```python
from build123d import *

# Parameters (mm, degrees)
SKETCH1_W           = 4
SKETCH1_H           = 15
BOSS_EXTRUDE1_DEPTH = 1
SKETCH2_R           = 1.5
CUT_EXTRUDE1_DEPTH  = 0.1
CUT_EXTRUDE2_DEPTH  = 0.2
SKETCH4_R           = 2.849028986
BOSS_EXTRUDE2_DEPTH = 4
CUT_EXTRUDE3_START  = -0.5
CUT_EXTRUDE3_DEPTH  = 3
SKETCH6_R           = 1
CUT_EXTRUDE4_DEPTH  = 50.5
BOSS_EXTRUDE3_REACH = 11.393
SKETCH7_W           = 4
SKETCH7_H           = 0.331547144
SKETCH8_R           = 1.5
BOSS_EXTRUDE4_DEPTH = 1.5
SKETCH13_R          = 2.5
CUT_EXTRUDE6_DEPTH  = 3
SKETCH14_R          = 1.5
BOSS_EXTRUDE5_DEPTH = 1
SKETCH15_R          = 1.65511662
CUT_EXTRUDE7_DEPTH  = 1.5
SKETCH16_W          = 5.099694499
SKETCH16_H          = 2.218752709
CUT_EXTRUDE8_DEPTH  = 3
FILLET1_R           = 0.2
SKETCH17_R          = 1.288740584
BOSS_EXTRUDE6_DEPTH = 1
FILLET2_R           = 1
SKETCH18_R          = 1.986595171
BOSS_EXTRUDE7_DEPTH = 0.5


with BuildPart() as part:
    # Sketch1 → Boss-Extrude1 (new body)
    with BuildSketch(Plane.XY):
        Rectangle(SKETCH1_W, SKETCH1_H)
    extrude(amount=BOSS_EXTRUDE1_DEPTH)

    # Sketch2 → Cut-Extrude1 (cut)
    with BuildSketch(Plane.XY.offset(1)):
        with Locations((0, -5.001272615)):
            Circle(SKETCH2_R)
        with Locations((0, -1.683913286)):
            Circle(SKETCH2_R)
    extrude(amount=-CUT_EXTRUDE1_DEPTH, mode=Mode.SUBTRACT)

    # Sketch3 → Cut-Extrude2 (cut)
    with BuildSketch(Plane.XY.offset(0.9)):
        Polygon((-0.108557852, -6.107102786), (0.108557852, -6.107102786), (0.108557852, -5.098298557), (0.933492592, -5.098298557), (0.933492592, -4.904246673), (0.108557852, -4.904246673), (0.108557852, -3.948637219), (-0.108557852, -3.948637219), (-0.108557852, -4.904246673), (-0.962043741, -4.904246673), (-0.962043741, -5.098298557), (-0.108557852, -5.098298557), align=None)
        Polygon((-0.962043741, -1.780939228), (-0.962043741, -1.586887344), (-0.108557852, -1.586887344), (-0.108557852, -0.578083116), (0.108557852, -0.578083116), (0.108557852, -1.586887344), (0.933492592, -1.586887344), (0.933492592, -1.780939228), (0.108557852, -1.780939228), (0.108557852, -2.736548682), (-0.108557852, -2.736548682), (-0.108557852, -1.780939228), align=None)
    extrude(amount=-CUT_EXTRUDE2_DEPTH, mode=Mode.SUBTRACT)

    # Sketch4 → Boss-Extrude2 (add)
    with BuildSketch(Plane(origin=(2, 0, 0), x_dir=(0, 0, -1), z_dir=(1, 0, 0))):
        with Locations((-2.871998104, 5.020758916)):
            Circle(SKETCH4_R)
    extrude(amount=-BOSS_EXTRUDE2_DEPTH)

    # Sketch5 → Cut-Extrude3 (cut)
    with BuildSketch(Plane(origin=(2, 0, 0), x_dir=(0, 0, -1), z_dir=(1, 0, 0)).offset(CUT_EXTRUDE3_START)):
        with BuildLine():
            Line((-2.871998104, 7.200015745), (-2.871998104, 9.297132531))
            Line((-2.871998104, 9.297132531), (-14.767112772, 7.450442617))
            Line((-14.767112772, 7.450442617), (-10.359701014, 0.939041163))
            Line((-10.359701014, 0.939041163), (-1.261981382, 2.30327176))
            Line((-1.261981382, 2.30327176), (-1.761184463, 3.145858016))
            ThreePointArc((-1.761184463, 3.145858016), (-0.770207092, 5.596636393), (-2.871998104, 7.200015745))
        make_face()
    extrude(amount=-CUT_EXTRUDE3_DEPTH, mode=Mode.SUBTRACT)

    # Sketch6 → Cut-Extrude4 (cut)
    with BuildSketch(Plane(origin=(2, 0, 0), x_dir=(0, 0, -1), z_dir=(1, 0, 0))):
        with Locations(Location((-2.871998104, 5.020758916, 0), (0, 0, 90))):
            Circle(SKETCH6_R)
    extrude(amount=-CUT_EXTRUDE4_DEPTH, mode=Mode.SUBTRACT)

    # Sketch7 → Boss-Extrude3 (add, up to next)
    with BuildSketch(Plane.XY.offset(1), mode=Mode.PRIVATE) as boss_extrude3_sk1:
        with Locations((0, 7.334226428)):
            Rectangle(SKETCH7_W, SKETCH7_H)
    boss_extrude3_tool1 = extrude(boss_extrude3_sk1.sketch, amount=BOSS_EXTRUDE3_REACH, mode=Mode.PRIVATE) - part.part
    add(boss_extrude3_tool1.solids().sort_by_distance((0, 7.334226, 1))[0])

    # Sketch8 → Boss-Extrude4 (add)
    with BuildSketch(Plane(origin=(0, 0, 0), x_dir=(-1, 0, 0), z_dir=(0, 0, -1))):
        with Locations(Location((0, -1.683913286, 0), (0, 0, 180))):
            Circle(SKETCH8_R)
        with Locations(Location((0, -5.001272615, 0), (0, 0, 180))):
            Circle(SKETCH8_R)
    extrude(amount=BOSS_EXTRUDE4_DEPTH)

    # Sketch13 → Cut-Extrude6 (cut)
    with BuildSketch(Plane(origin=(-1.5, 0, 0), x_dir=(0, 0, -1), z_dir=(1, 0, 0))):
        with Locations((-2.871998104, 5.020758916)):
            Circle(SKETCH13_R)
    extrude(amount=CUT_EXTRUDE6_DEPTH, mode=Mode.SUBTRACT)

    # Sketch14 → Boss-Extrude5 (add)
    with BuildSketch(Plane.XY.offset(1)):
        with Locations((0, -5.001272615)):
            Circle(SKETCH14_R)
    extrude(amount=-BOSS_EXTRUDE5_DEPTH)

    # Sketch15 → Cut-Extrude7 (cut)
    with BuildSketch(Plane(origin=(0, 0, -1.5), x_dir=(-1, 0, 0), z_dir=(0, 0, -1))):
        with Locations((0, -5.001272615)):
            Circle(SKETCH15_R)
    extrude(amount=-CUT_EXTRUDE7_DEPTH, mode=Mode.SUBTRACT)

    # Sketch16 → Cut-Extrude8 (cut)
    with BuildSketch(Plane.XZ.offset(7.5)):
        with Locations((0.205566766, 0.392687456)):
            Rectangle(SKETCH16_W, SKETCH16_H)
    extrude(amount=-CUT_EXTRUDE8_DEPTH, mode=Mode.SUBTRACT)

    # Fillet1
    fillet1_edges = [part.edges().sort_by_distance(p)[0] for p in [
        (0, 7.869787902, 2.871998104),
        (2, 4.733861171, 5.706544954),
        (0, 7.5, 1.468313735),
        (2, -0.813467512, 1),
        (-2, -4.5, 0.5),
        (2, -4.5, 0.5),
        (0, -4.5, 1),
        (-2, 7.5, 0.734156868),
        (2, 7.5, 0.734156868),
        (-2, -0.813467512, 1),
        (0, 2.873064976, 1),
        (-2, 4.733861171, 5.706544954),
    ]]
    fillet(fillet1_edges, radius=FILLET1_R)

    # Sketch17 → Boss-Extrude6 (add)
    with BuildSketch(Plane(origin=(0, 0, 0), x_dir=(-1, 0, 0), z_dir=(0, 0, -1))):
        with Locations(Location((0, 4.363041625, 0), (0, 0, 180))):
            Circle(SKETCH17_R)
    extrude(amount=BOSS_EXTRUDE6_DEPTH)

    # Fillet2
    fillet2_edges = [part.edges().sort_by_distance(p)[0] for p in [
        (-1.288740584, 4.363041625, -1),
    ]]
    fillet(fillet2_edges, radius=FILLET2_R - 0.0001)  # a hair under: the kernel refuses the full size

    # Sketch18 → Boss-Extrude7 (add)
    with BuildSketch(Plane(origin=(0, 0, -1.5), x_dir=(-1, 0, 0), z_dir=(0, 0, -1))):
        with Locations((0, -1.683913286)):
            Circle(SKETCH18_R)
    extrude(amount=-BOSS_EXTRUDE7_DEPTH)


solid = part.part
```
The model under review builds one solid part; all positions refer to its coordinate system, in mm. A direction names the side the tool comes from. Round coordinates to 2 decimals unless told otherwise and drop trailing zeros. Loops run counter-clockwise (first coordinate to the right, second up) from the corner with the lowest first, then second, coordinate; pieces in that order, holes last. Notation, with made-up numbers: (46.5, -4) -> (91.5, -4) arc R14 cw to (91.5, 16) -> close; hole circle Ø7 at (70, -30). An arc over 180 degrees is marked (long way). Answer as a JSON object with one key per item and string values. Group by question number.
1) For faces 4 (the face through (2, 4, 2)), 5 (the face through (0, 0, -1)), 6 (the face through (0, 7.5, 1)), 7 (the face through (0.3, -2, 0.9)), list the 3-axis set-ups (+Z, -Z, +X, -X, +Y, -Y) from which the entire face can be reached by the end or side of a thin tool; tool diameter is ignored.
2) For pin 1 Ø1.1 at (x, y) = (-0.5, -1.5) entering from +Z, flat-tipped, find the tip position at first contact; note if it passes through.
3) Mouldability with a two-part tool opening along Y and no side actions: class faces 1 (the face through (-2, 4, 2)), 2 (the face through (-1.9, -1.1, -1.3)), 3 (the face through (-0.33, -0.22, -0.49)) as released by +Y, released by -Y, zero draft, split by the parting line, or undercut.
4) We need section A-A on y = 2. Write out the cut boundary in (x, z), then the cut area to 3 significant figures.
5) We need section B-B on z = 3.25. Give the number of separate pieces and of enclosed holes in the cut face, then the cut area to 3 significant figures.
6) For line 1 (X direction, y = 3.75, z = 0.75); line 2 (Z direction, x = -1.15, y = -0.5); line 3 (Z direction, x = -0.6, y = -1.5), list the stretches that pass through material, from the lowest coordinate up. Write a range as [from, to].
Result set:
{
 "1": {"face 4": "+Z, -Z, +X, +Y, -Y", "face 5": "none", "face 6": "-Z, +X, -X, +Y", "face 7": "+Z"},
 "2": {"pin 1": "z = 0.9"},
 "3": {"face 1": "zero draft", "face 2": "split by the parting line", "face 3": "undercut"},
 "4": {"outline": "(-2, 0) -> (2, 0) -> (2, 0.8) arc R0.2 ccw to (1.8, 1) -> (-1.8, 1) arc R0.2 ccw to (-2, 0.8) -> close", "area": "3.98 mm²"},
 "5": {"separate pieces": "4", "enclosed holes": "0", "area": "3.76 mm²"},
 "6": {"line 1": "[-2, -1.5], [1.5, 2]", "line 2": "[-1.5, -1], [0, 1]", "line 3": "[-1.5, 0.9]"}
}
